Check sheet for the modelled part. Datum: model origin and axes. Units: mm. Face numbers are marked on the shaded views. Give positions to 0.01 mm unless a question says otherwise; leave off trailing zeros. Loops run counter-clockwise (first coordinate to the right, second up) from the corner with the lowest first, then second, coordinate; pieces in that order, holes last. Notation, with made-up numbers: (22, 51.5) -> (53, 51.5) arc R8 cw to (53, 60.5) -> close; hole circle Ø2 at (-5, 37.25). An arc over 180 degrees is marked (long way). Write each question's results on one line, items separated by ' | '. Start each with the question number.
1. Gauge pin test, flat ends, axial feed: pin 1 Ø1.5 at (y, z) = (-7, 12) entering from +X; pin 2 Ø1.5 at (x, y) = (6.5, -10) entering from -Z; pin 3 Ø4 at (y, z) = (-13.5, 11) entering from +X. Record the tip position at first contact, or that the pin passes through.
2. Material ranges on L1, parallel to Z at x = 7.5, y = -9.25; L2, parallel to Z at x = 10.25, y = -11; L3, parallel to Z at x = 13, y = -5.75, recorded low to high. Write a range as from..to.
3. Cross-section at D-D on z = -9. Record the boundary of the cut face in (x, y), and give its area (3 significant figures).
4. Cross-section at A-A on y = -14.5. Record the boundary of the cut face in (x, z), and give its area (3 significant figures).
5. Mould release check, pull along X, two halves, no side actions. Record for the marked faces 1, 2 and 3: +X half, -X half, draft (parallel to the pull), parting line (faces both ways), or undercut.
6. Cross-section at C-C on y = -16.5. Record the boundary of the cut face in (x, z), and give its area (3 significant figures).
7. Cross-section at B-B on z = 0. Record the boundary of the cut face in (x, y), and give its area (3 significant figures).
from build123d import *

# Parameters (mm, degrees)
SKETCH_R    = 5
PAD_DEPTH   = 18
FILLET_R    = 8
FILLET001_R = 10
FILLET002_R = 2


with BuildPart() as part:
    # Sketch → Pad (new body)
    with BuildSketch(Plane.XZ):
        Polygon((4, 17.5), (0, 17.5), (0, -17.5), (4, -17.5), (4, -12.5), (19.5, 0), (4, 12.5), align=None)
        with Locations((7.5, 0)):
            Circle(SKETCH_R, mode=Mode.SUBTRACT)
    extrude(amount=PAD_DEPTH)

    # Fillet
    fillet_edges = [part.edges().sort_by_distance(p)[0] for p in [
        (19.5, -9, 0),
    ]]
    fillet(fillet_edges, radius=FILLET_R)

    # Fillet001
    fillet001_edges = [part.edges().sort_by_distance(p)[0] for p in [
        (4, -9, -12.5),
        (4, -9, 12.5),
    ]]
    fillet(fillet001_edges, radius=FILLET001_R)

    # Fillet002
    fillet002_edges = [part.edges().sort_by_distance(p)[0] for p in [
        (2.5, -18, 0),
        (2.5, 0, 0),
    ]]
    fillet(fillet002_edges, radius=FILLET002_R)


solid = part.part
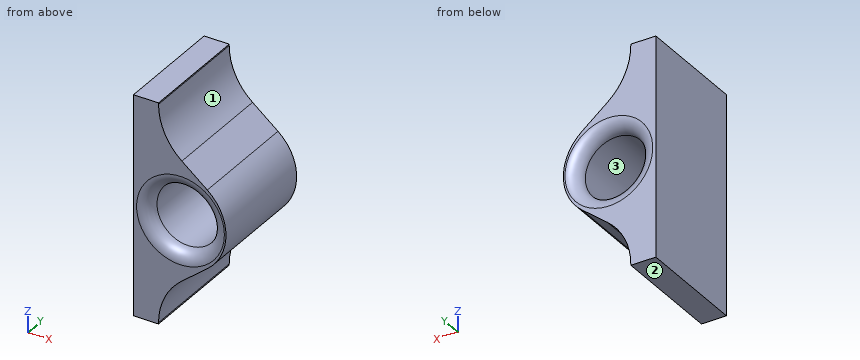
Geometry says:
1) pin 1: x = 6.02 | pin 2: z = -11.63 | pin 3: x = 8.34
2) L1: -9.68..-5, 5..9.68 | L2: -7.46..-4.18, 4.18..7.46 | L3: -5..5
3) outline: (0, -18) -> (8.34, -18) -> (8.34, 0) -> (0, 0) -> close | area: 150 mm^2
4) outline: (0, -17.5) -> (4, -17.5) -> (4, -17.28) arc R10 cw to (7.72, -9.5) -> (11.78, -6.23) arc R8 ccw to (11.78, 6.23) -> (7.72, 9.5) arc R10 cw to (4, 17.28) -> (4, 17.5) -> (0, 17.5) -> close; hole circle Ø10 at (7.5, 0) | area: 239 mm^2
5) face 1: +X half | face 2: draft | face 3: undercut
6) outline: (0, -17.5) -> (4, -17.5) -> (4, -17.28) arc R10 cw to (7.72, -9.5) -> (11.78, -6.23) arc R8 ccw to (11.78, 6.23) -> (7.72, 9.5) arc R10 cw to (4, 17.28) -> (4, 17.5) -> (0, 17.5) -> close; hole circle Ø10.13 at (7.5, 0) | area: 237 mm^2
7) outline: (0, -18) -> (0.5, -18) arc R2 ccw to (2.5, -16) -> (2.5, -2) arc R2 ccw to (0.5, 0) -> (0, 0) -> close; (12.5, -16) arc R2 ccw to (14.5, -18) -> (14.76, -18) -> (14.76, 0) -> (14.5, 0) arc R2 ccw to (12.5, -2) -> close | area: 82.2 mm^2
